```python
from build123d import *

# Parameters (mm, degrees)
SKETCH_1_R          = 24.5
EXTRUDE_1_DEPTH     = 18
FILLET_1_R          = 1
SKETCH_2_R          = 24.5
EXTRUDE_2_DEPTH     = 21
CHAMFER_1_SIZE      = 1
CHAMFER_2_SIZE      = 1
SKETCH_4_R          = 6.3
CUT_EXTRUDE_1_DEPTH = 10
SKETCH_5_R          = 1.5
CUT_EXTRUDE_2_DEPTH = 5
SKETCH_6_R          = 1.5
CUT_EXTRUDE_3_DEPTH = 5


with BuildPart() as part:
    # 草图1 → 凸台-拉伸1 (new body)
    with BuildSketch(Plane(origin=(0, 0, 0), x_dir=(1, 0, 0), z_dir=(0, 1, 0))):
        Circle(SKETCH_1_R)
    extrude(amount=EXTRUDE_1_DEPTH)

    # 圆角1
    fillet_1_edges = [part.edges().sort_by_distance(p)[0] for p in [
        (-24.5, 18, 0),
    ]]
    fillet(fillet_1_edges, radius=FILLET_1_R)

    # 草图2 → 凸台-拉伸2 (add)
    with BuildSketch(Plane(origin=(0, 18, 0), x_dir=(1, 0, 0), z_dir=(0, 1, 0))):
        Circle(SKETCH_2_R)
    extrude(amount=EXTRUDE_2_DEPTH)

    # 倒角1
    chamfer_1_edges = [part.edges().sort_by_distance(p)[0] for p in [
        (-24.5, 39, 0),
    ]]
    chamfer(chamfer_1_edges, length=CHAMFER_1_SIZE)

    # 倒角2
    chamfer_2_edges = [part.edges().sort_by_distance(p)[0] for p in [
        (-24.5, 0, 0),
    ]]
    chamfer(chamfer_2_edges, length=CHAMFER_2_SIZE)

    # 草图4 → 切除-拉伸1 (cut)
    with BuildSketch(Plane(origin=(0, 39, 0), x_dir=(1, 0, 0), z_dir=(0, 1, 0))):
        Circle(SKETCH_4_R)
    extrude(amount=-CUT_EXTRUDE_1_DEPTH, mode=Mode.SUBTRACT)

    # 草图5 → 切除-拉伸2 (cut)
    with BuildSketch(Plane(origin=(0, 39, 0), x_dir=(1, 0, 0), z_dir=(0, 1, 0))):
        with Locations((9.5, 0)):
            Circle(SKETCH_5_R)
        with Locations((0, -9.5)):
            Circle(SKETCH_5_R)
        with Locations((-9.5, 0)):
            Circle(SKETCH_5_R)
        with Locations((0, 9.5)):
            Circle(SKETCH_5_R)
        with Locations((8.838834765, 8.838834765)):
            Circle(SKETCH_5_R)
        with Locations((8.838834765, -8.838834765)):
            Circle(SKETCH_5_R)
        with Locations((-8.838834765, -8.838834765)):
            Circle(SKETCH_5_R)
        with Locations((-8.838834765, 8.838834765)):
            Circle(SKETCH_5_R)
    extrude(amount=-CUT_EXTRUDE_2_DEPTH, mode=Mode.SUBTRACT)

    # 草图6 → 切除-拉伸3 (cut)
    with BuildSketch(Plane.XZ):
        with Locations((15, 0)):
            Circle(SKETCH_6_R)
        with Locations((0, -15)):
            Circle(SKETCH_6_R)
        with Locations((-15, 0)):
            Circle(SKETCH_6_R)
        with Locations((0, 15)):
            Circle(SKETCH_6_R)
    extrude(amount=-CUT_EXTRUDE_3_DEPTH, mode=Mode.SUBTRACT)


solid = part.part
```
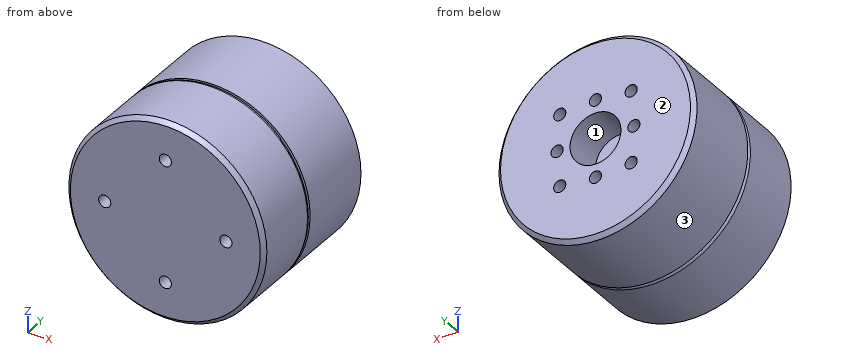
Source: CAD feature listing. Evaluate the final solid. Frame: model axes, mm. Face numbers are marked on the shaded views. Round coordinates to 2 decimals unless told otherwise and drop trailing zeros. Write each loop counter-clockwise with the first axis right and the second up, starting at its lowest first coordinate (ties: lowest second). Pieces come first, ordered by that corner, then holes. Notation, with made-up numbers: M 44,-22 L 60,-22 A29 ccw 60,11 Z; hole C 31,-37.5 d2. An arc over 180 degrees is marked long. Answer as a JSON object with one key per item and string values. Group by question number.
(1) Mould query, pull axis Z, two halves, no side actions, for the marked faces 1, 2 and 3. Classes: +Z half, -Z half, draft (parallel to the pull), parting line (faces both ways), or undercut.
(2) Ray query, line 1 (X direction, y = 35.5, z = 0); line 2 (X direction, y = 33, z = 0). Return the intervals inside material, ascending. Write a range as [from, to].
(3) Section query B-B on y = 11. Output: boundary loops of the cut face in (x, z).
(4) First-contact query: pin 1 (0.9 mm diameter, centred on x = 15, z = 0.5, fed in from -Y); pin 2 (5 mm diameter, centred on x = 19.5, z = -18.5, fed in from -Y); pin 3 (1.5 mm diameter, centred on x = 0, z = -9, fed in from +Y). Flat tips, straight axial feed; report the tip coordinate or a pass-through.
Computed values:
{
 "1": {"face 1": "undercut", "face 2": "draft", "face 3": "parting line"},
 "2": {"line 1": "[-24.5, -11], [-8, -6.3], [6.3, 8], [11, 24.5]", "line 2": "[-24.5, -6.3], [6.3, 24.5]"},
 "3": {"outline": "C 0,0 d49"},
 "4": {"pin 1": "y = 5", "pin 2": "y = 0.88", "pin 3": "y = 34"}
}
